from build123d import *

# Parameters (mm, degrees)
F0_W     = 5
F0_H     = 10
F0_W_2   = 20.5440539549
F2_SIZE  = 5
F3_DEPTH = 100


with BuildPart() as f1:
    # F0 (on Front) → F1 (revolve)
    with BuildSketch(Plane.XZ):
        Polygon((12.7720269775, 5), (12.7720269775, -5), (7.7720269775, -5), (7.7720269775, -12.5), (17.7720269775, -12.5), (17.7720269775, 12.5), (7.7720269775, 12.5), (7.7720269775, 5), align=None)
        with Locations((10.2720269775, 0)):
            Rectangle(F0_W, F0_H)
        with Locations((-2.5, 0)):
            Rectangle(F0_W_2, F0_H)
    revolve(axis=Axis((12.7720269775, 0, 12.5), (-1, 0, 0)))

    # F2
    f2_edges = [f1.edges().sort_by_distance(p)[0] for p in [
        (7.772027, 0, 37.5),
    ]]
    chamfer(f2_edges, length=F2_SIZE)

    # F3 (add): a face of the model
    f3_faces = [f1.faces().sort_by_distance(p)[0] for p in [
        (-12.7720269775, 0, 20.4949747468),
    ]]
    extrude(f3_faces, amount=F3_DEPTH)


solid = f1.part
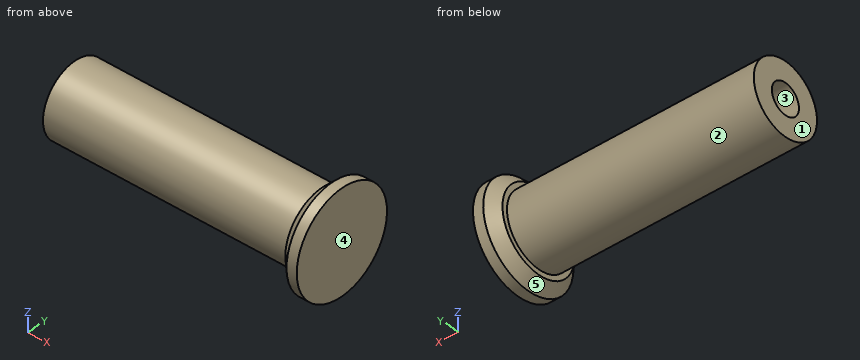
Read the model definition and answer for the solid it produces. Units are mm, in the model's axes. Face numbers are marked on the shaded views. A direction names the side the tool comes from. Coordinates: 2 decimals unless noted, no trailing zeros. Order: outer loops, then holes, each group sorted by start corner. A loop starts at its lowest first (then second) coordinate and runs counter-clockwise, first axis right, second up. Notation, with made-up numbers: (58, 11) -> (117, 11) arc R16 ccw to (117, 31) -> close; hole circle Ø2 at (47, -7.75). An arc over 180 degrees is marked (long way). Answer as a JSON object with one key per item and string values.
1) A cutting plane is placed at C-C, the plane x = -2. Determine the outline of the cut face in (y, z), plus the area to 3 significant figures.
Model answer:
{"outline": "circle Ø35 at (0, 12.5); hole circle Ø15 at (0, 12.5)", "area": "785 mm²"}
2) The mould has two halves that part along Y. Classify the marked faces 3, 4 and 5: released by +Y, released by -Y, zero draft, split by the parting line, or undercut.
Model answer:
{"face 3": "undercut", "face 4": "zero draft", "face 5": "split by the parting line"}
3) Each of these flat-tipped pins is pushed along its axis until it touches: pin 1 (12 mm diameter, centred on y = 18, z = 27.5, fed in from -X); pin 2 (6 mm diameter, centred on x = -84.5, y = 11.5, fed in from -Z); pin 3 (1.5 mm diameter, centred on x = -42.5, z = 31.5, fed in from +Y); pin 4 (1.5 mm diameter, centred on x = -43, y = -0.5, fed in from +Z). Where does it stop, or does it pass through?
Model answer:
{"pin 1": "stops at x = -112.77", "pin 2": "stops at z = -2.8", "pin 3": "passes through", "pin 4": "stops at z = 30"}
4) A cutting plane is placed at A-A, the plane y = 0. Determine the outline of the cut face in (x, z), plus the area to 3 significant figures.
Model answer:
{"outline": "(-112.77, -5) -> (7.77, -5) -> (7.77, -7.5) -> (12.77, -12.5) -> (17.77, -12.5) -> (17.77, 37.5) -> (12.77, 37.5) -> (7.77, 32.5) -> (7.77, 30) -> (-112.77, 30) -> (-112.77, 20) -> (7.77, 20) -> (7.77, 5) -> (-112.77, 5) -> close", "area": "2,890 mm²"}
5) Consider line 1 along Z through (x, y) = (-49, 0); line 2 along Y through (x, z) = (-87.5, 12.5); line 3 along X through (y, z) = (5, 8.5). Determine where each line is inside the solid, lowest interval first. Write a range as from..to.
Model answer:
{"line 1": "z = -5..5, 20..30", "line 2": "y = -17.5..-7.5, 7.5..17.5", "line 3": "x = 7.77..17.77"}
6) A tool of negligible diameter and unlimited length cuts with its end or side. For the marked faces 1 and 2, from which of +Z, -Z, +X, -X, +Y, -Y can it reach the whole face along a straight path? Write none if from no direction.
Model answer:
{"face 1": "+Z, -Z, -X, +Y, -Y", "face 2": "-X"}
7) A cutting plane is placed at B-B, the plane z = 12.5. Determine the outline of the cut face in (x, y).
Model answer:
{"outline": "(-112.77, -17.5) -> (7.77, -17.5) -> (7.77, -20) -> (12.77, -25) -> (17.77, -25) -> (17.77, 25) -> (12.77, 25) -> (7.77, 20) -> (7.77, 17.5) -> (-112.77, 17.5) -> (-112.77, 7.5) -> (7.77, 7.5) -> (7.77, -7.5) -> (-112.77, -7.5) -> close"}
